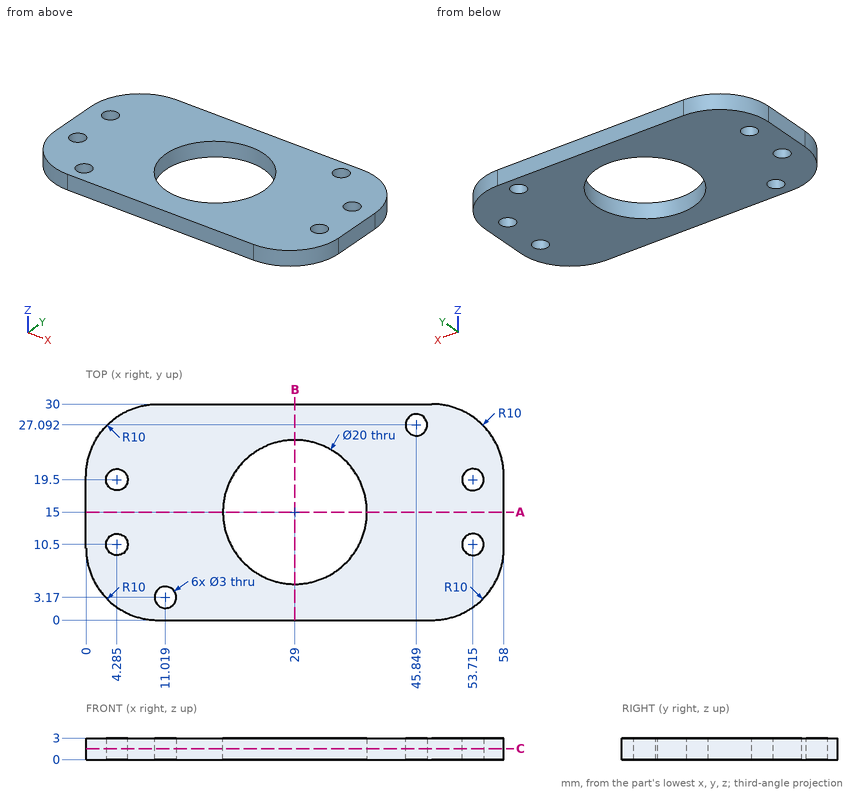
The figure shows three views and two pictorial views of one solid part (mm, origin at its lowest corner). Answer the questions. Round coordinates to 2 decimals unless told otherwise and drop trailing zeros. Loops run counter-clockwise (first coordinate to the right, second up) from the corner with the lowest first, then second, coordinate; pieces in that order, holes last. Notation, with made-up numbers: (77, -1.75) -> (134, -1.75) arc R19 cw to (134, 21.25) -> close; hole circle Ø7 at (-24, 74). An arc over 180 degrees is marked (long way). Use one line per item in the form item = value.
(1) Straight lines are drawn through the part: line 1 (X direction, y = 14.5, z = 2.1); line 2 (Y direction, x = 29, z = 1.1); line 3 (X direction, y = 10.75, z = 1.85) (1 decimal). For each, find the intervals that lie inside material, in ascending order.
Answer list:
line_1 = 0 to 19.01, 38.99 to 58
line_2 = 0 to 5, 25 to 30
line_3 = 0 to 2.8, 5.8 to 19.9, 38.1 to 52.2, 55.2 to 58
(2) Find section C-C on z = 1.55. Give the number of separate pieces and of enclosed holes in the cut face, then the cut area to 3 significant figures.
Answer list:
separate_pieces = 1
enclosed_holes = 7
area = 1,300 mm2
(3) Flat-ended cylindrical pins translate along their axes: P1, Ø4, axis at x = 11.02, y = 3.17, coming from the -Z side; P2, Ø12, axis at x = 29, y = 15, coming from the +Z side; P3, Ø1.5, axis at y = 6.5, z = 1, coming from the +X side (1 decimal). Find the tip coordinate at first contact, or state that the pin passes through.
Answer list:
P1 = 0
P2 = through
P3 = 57.6
(4) Find section A-A on y = 15. Give the vertices of the cut face in (x, z), then the cut area to 3 significant figures.
Answer list:
outline = (0, 0) -> (19, 0) -> (19, 3) -> (0, 3) -> close; (39, 0) -> (58, 0) -> (58, 3) -> (39, 3) -> close
area = 114 mm2
(5) Find section B-B on x = 29. Give the vertices of the cut face in (y, z), then the cut area to 3 significant figures.
Answer list:
outline = (0, 0) -> (5, 0) -> (5, 3) -> (0, 3) -> close; (25, 0) -> (30, 0) -> (30, 3) -> (25, 3) -> close
area = 30.0 mm2
